Check sheet for the modelled part. Datum: model origin and axes. Units: mm. Round coordinates to 2 decimals unless told otherwise and drop trailing zeros. Loops run counter-clockwise (first coordinate to the right, second up) from the corner with the lowest first, then second, coordinate; pieces in that order, holes last. Notation, with made-up numbers: (29, 74) -> (48, 74) arc R23 cw to (48, 90) -> close; hole circle Ø6 at (-27.75, 18.5). An arc over 180 degrees is marked (long way). Use one line per item in the form item = value. Start each with the question number.
(1) Go/stop test with flat-tipped pins: pin 1 (2 mm diameter, centred on x = 8, y = -18.5, fed in from -Z); pin 2 (1.5 mm diameter, centred on y = -20, z = 96.5, fed in from +X). Record where each tip stops, or that it passes through.
(2) Sectioned sample at C-C (z = 220.5). Record the cut outline in (x, y), and give its area (3 significant figures).
(3) Sectioned sample at B-B (x = 26.5). Record the cut outline in (y, z), and give its area (3 significant figures).
(4) Sectioned sample at A-A (y = -14.75). Record the cut outline in (x, z), and give its area (3 significant figures).
(5) Material ranges on probe 1 along Z at (x, y) = (-54.5, -10.25); probe 2 along X at (y, z) = (-9, 159.5); probe 3 along X at (y, z) = (-9.75, 160), recorded low to high. Write a range as [from, to].
from build123d import *

# Parameters (mm, degrees)
F1_DEPTH = 25.4


with BuildPart() as f1:
    # F0 (on Front) → F1 (new body)
    with BuildSketch(Plane.XZ):
        with BuildLine():
            Line((-113.4872, 0), (-109.0422, 0))
            Line((-109.0422, 0), (0, 0))
            Line((0, 0), (67.239726, 111.464568))
            Line((67.239726, 111.464568), (44.77097, 160.540587))
            ThreePointArc((44.77097, 160.540587), (1.021835, 205.134265), (-16.943187, 264.966037))
            ThreePointArc((-16.943187, 264.966037), (-45.82596, 194.637581), (-109.0422, 152.4))
            Line((-109.0422, 152.4), (-113.4872, 0))
        make_face()
    extrude(amount=F1_DEPTH)


solid = f1.part
Checks:
q1.pin_1 = 11.6
q1.pin_2 = 58.66
q2.outline = (-29.33, -25.4) -> (-6.74, -25.4) -> (-6.74, 0) -> (-29.33, 0) -> close
q2.area = 574 mm2
q3.outline = (-25.4, 43.93) -> (0, 43.93) -> (0, 174.16) -> (-25.4, 174.16) -> close
q3.area = 3,310 mm2
q4.outline = (-113.49, 0) -> (0, 0) -> (67.24, 111.46) -> (44.77, 160.54) arc R130.3 cw to (-16.94, 264.97) arc R130.3 cw to (-109.04, 152.4) -> close
q4.area = 28,600 mm2
q5.probe_1 = [0, 185.05]
q5.probe_2 = [-90.66, 45.25]
q5.probe_3 = [-89.63, 45.02]
